Model file for the job. Use its own axes, mm. A direction names the side the tool comes from. Coordinates: 2 decimals unless noted, no trailing zeros. Order: outer loops, then holes, each group sorted by start corner. A loop starts at its lowest first (then second) coordinate and runs counter-clockwise, first axis right, second up.
from build123d import *

# Parameters (mm, degrees)
SKETCH1_R                                        = 28.448
EXTRUDE1_DEPTH                                   = 7.9375
CBORE_FOR_1_4_SOCKET_HEAD_CAP_SCREW1_D           = 6.7564
CBORE_FOR_1_4_SOCKET_HEAD_CAP_SCREW1_DEPTH       = 9.525
CBORE_FOR_1_4_SOCKET_HEAD_CAP_SCREW1_CBORE_D     = 11.1125
CBORE_FOR_1_4_SOCKET_HEAD_CAP_SCREW1_CBORE_DEPTH = 6.35
F_1_4_20_TAPPED_HOLE1_D                          = 5.1054
CBORE_FOR_1_4_SOCKET_HEAD_CAP_SCREW3_D           = 6.7564
CBORE_FOR_1_4_SOCKET_HEAD_CAP_SCREW3_DEPTH       = 9.525
CBORE_FOR_1_4_SOCKET_HEAD_CAP_SCREW3_CBORE_D     = 11.1125
CBORE_FOR_1_4_SOCKET_HEAD_CAP_SCREW3_CBORE_DEPTH = 6.35
F_1_4_20_TAPPED_HOLE4_D                          = 5.1054
CBORE_FOR_1_4_SOCKET_HEAD_CAP_SCREW4_D           = 6.7564
CBORE_FOR_1_4_SOCKET_HEAD_CAP_SCREW4_DEPTH       = 9.525
CBORE_FOR_1_4_SOCKET_HEAD_CAP_SCREW4_CBORE_D     = 11.1125
CBORE_FOR_1_4_SOCKET_HEAD_CAP_SCREW4_CBORE_DEPTH = 6.35
F_1_4_20_TAPPED_HOLE5_D                          = 5.1054
F_1_4_20_TAPPED_HOLE5_DEPTH                      = 9.525
CBORE_FOR_1_4_SOCKET_HEAD_CAP_SCREW5_D           = 6.7564
CBORE_FOR_1_4_SOCKET_HEAD_CAP_SCREW5_DEPTH       = 9.525
CBORE_FOR_1_4_SOCKET_HEAD_CAP_SCREW5_CBORE_D     = 11.1125
CBORE_FOR_1_4_SOCKET_HEAD_CAP_SCREW5_CBORE_DEPTH = 6.35
F_1_4_20_TAPPED_HOLE6_D                          = 5.1054
F_1_4_20_TAPPED_HOLE6_DEPTH                      = 9.525
FILLET1_R                                        = 3.175


with BuildPart() as part:
    # Sketch1 → Extrude1 (new, symmetric)
    with BuildSketch(Plane.XY):
        with BuildLine():
            Line((-39.6875, 76.2), (-39.6875, 0))
            ThreePointArc((-39.6875, 0), (-32.485618813, -22.798733003), (-13.49375, -37.323134477))
            Line((-13.49375, -37.323134477), (-13.49375, -56.373134477))
            Line((-13.49375, -56.373134477), (-3.96875, -56.373134477))
            Line((-3.96875, -56.373134477), (-3.96875, -36.296166184))
            ThreePointArc((-3.96875, -36.296166184), (0, 36.5125), (3.96875, -36.296166184))
            Line((3.96875, -36.296166184), (3.96875, -56.373134477))
            Line((3.96875, -56.373134477), (13.49375, -56.373134477))
            Line((13.49375, -56.373134477), (13.49375, -37.323134477))
            ThreePointArc((13.49375, -37.323134477), (15.940663019, -36.345466275), (18.317307692, -35.207582921))
            Line((18.317307692, -35.207582921), (46.483374029, -20.553736767))
            Line((46.483374029, -20.553736767), (55.275681722, -37.45337657))
            Line((55.275681722, -37.45337657), (63.725501623, -33.057222723))
            Line((63.725501623, -33.057222723), (54.93319393, -16.157582921))
            Line((54.93319393, -16.157582921), (31.487040084, 28.908123218))
            ThreePointArc((31.487040084, 28.908123218), (33.176067607, 34.260612279), (38.528556668, 32.571584756))
            Line((38.528556668, 32.571584756), (61.974710515, -12.494121383))
            Line((61.974710515, -12.494121383), (70.767018207, -29.393761185))
            Line((70.767018207, -29.393761185), (79.216838108, -24.997607339))
            Line((79.216838108, -24.997607339), (70.424530416, -8.097967537))
            Line((70.424530416, -8.097967537), (91.549080168, 2.892417079))
            ThreePointArc((91.549080168, 2.892417079), (112.919272476, 38.1), (91.549080168, 73.307582921))
            Line((91.549080168, 73.307582921), (70.424530416, 84.297967537))
            Line((70.424530416, 84.297967537), (79.216838108, 101.197607339))
            Line((79.216838108, 101.197607339), (70.767018207, 105.593761185))
            Line((70.767018207, 105.593761185), (61.974710515, 88.694121383))
            Line((61.974710515, 88.694121383), (38.528556668, 43.628415244))
            ThreePointArc((38.528556668, 43.628415244), (33.176067607, 41.939387721), (31.487040084, 47.291876782))
            Line((31.487040084, 47.291876782), (54.93319393, 92.357582921))
            Line((54.93319393, 92.357582921), (63.725501623, 109.257222723))
            Line((63.725501623, 109.257222723), (55.275681722, 113.65337657))
            Line((55.275681722, 113.65337657), (46.483374029, 96.753736767))
            Line((46.483374029, 96.753736767), (18.317307692, 111.407582921))
            ThreePointArc((18.317307692, 111.407582921), (15.940663019, 112.545466275), (13.49375, 113.523134477))
            Line((13.49375, 113.523134477), (13.49375, 132.573134477))
            Line((13.49375, 132.573134477), (3.96875, 132.573134477))
            Line((3.96875, 132.573134477), (3.96875, 112.496166184))
            ThreePointArc((3.96875, 112.496166184), (0, 39.6875), (-3.96875, 112.496166184))
            Line((-3.96875, 112.496166184), (-3.96875, 132.573134477))
            Line((-3.96875, 132.573134477), (-13.49375, 132.573134477))
            Line((-13.49375, 132.573134477), (-13.49375, 113.523134477))
            ThreePointArc((-13.49375, 113.523134477), (-32.485618813, 98.998733003), (-39.6875, 76.2))
        make_face()
        with Locations((73.231772476, 38.1)):
            Circle(SKETCH1_R, mode=Mode.SUBTRACT)
    extrude(amount=EXTRUDE1_DEPTH, both=True)

    # CBORE for 1/4 Socket Head Cap Screw1
    with Locations(Plane(origin=(13.49375, 0, 0), x_dir=(0, 0, -1), z_dir=(1, 0, 0))):
        with Locations((0, 123.048134477)):
            CounterBoreHole(CBORE_FOR_1_4_SOCKET_HEAD_CAP_SCREW1_D / 2, CBORE_FOR_1_4_SOCKET_HEAD_CAP_SCREW1_CBORE_D / 2, CBORE_FOR_1_4_SOCKET_HEAD_CAP_SCREW1_CBORE_DEPTH, depth=CBORE_FOR_1_4_SOCKET_HEAD_CAP_SCREW1_DEPTH)

    # 1/4-20 Tapped Hole1 (through all)
    with Locations(Plane(origin=(-3.96875, 0, 0), x_dir=(0, 0, -1), z_dir=(1, 0, 0))):
        with Locations((0, 123.048134477)):
            Hole(F_1_4_20_TAPPED_HOLE1_D / 2)

    # CBORE for 1/4 Socket Head Cap Screw3
    with Locations(Plane(origin=(13.49375, 0, 0), x_dir=(0, 0, -1), z_dir=(1, 0, 0))):
        with Locations((0, -46.848134477)):
            CounterBoreHole(CBORE_FOR_1_4_SOCKET_HEAD_CAP_SCREW3_D / 2, CBORE_FOR_1_4_SOCKET_HEAD_CAP_SCREW3_CBORE_D / 2, CBORE_FOR_1_4_SOCKET_HEAD_CAP_SCREW3_CBORE_DEPTH, depth=CBORE_FOR_1_4_SOCKET_HEAD_CAP_SCREW3_DEPTH)

    # 1/4-20 Tapped Hole4 (through all)
    with Locations(Plane(origin=(-3.96875, 0, 0), x_dir=(0, 0, -1), z_dir=(1, 0, 0))):
        with Locations((0, -46.848134477)):
            Hole(F_1_4_20_TAPPED_HOLE4_D / 2)

    # CBORE for 1/4 Socket Head Cap Screw4
    with Locations(Plane(origin=(20.907887704, -10.877662722, 0), x_dir=(0, 0, -1), z_dir=(0.8871201995900625, -0.46153846153845923, 0))):
        with Locations((0, 116.811059209)):
            CounterBoreHole(CBORE_FOR_1_4_SOCKET_HEAD_CAP_SCREW4_D / 2, CBORE_FOR_1_4_SOCKET_HEAD_CAP_SCREW4_CBORE_D / 2, CBORE_FOR_1_4_SOCKET_HEAD_CAP_SCREW4_CBORE_DEPTH, depth=CBORE_FOR_1_4_SOCKET_HEAD_CAP_SCREW4_DEPTH)

    # 1/4-20 Tapped Hole5
    with Locations(Plane(origin=(5.416551219, -2.818047337, 0), x_dir=(0, 0, -1), z_dir=(0.8871201995900618, -0.4615384615384606, 0))):
        with Locations((0, 116.811059209)):
            Hole(F_1_4_20_TAPPED_HOLE5_D / 2, depth=F_1_4_20_TAPPED_HOLE5_DEPTH)

    # CBORE for 1/4 Socket Head Cap Screw5
    with Locations(Plane(origin=(52.107222723, 27.109615385, 0), x_dir=(0, 0, -1), z_dir=(0.8871201995900624, 0.46153846153845934, 0))):
        with Locations((0, -49.2125)):
            CounterBoreHole(CBORE_FOR_1_4_SOCKET_HEAD_CAP_SCREW5_D / 2, CBORE_FOR_1_4_SOCKET_HEAD_CAP_SCREW5_CBORE_D / 2, CBORE_FOR_1_4_SOCKET_HEAD_CAP_SCREW5_CBORE_DEPTH, depth=CBORE_FOR_1_4_SOCKET_HEAD_CAP_SCREW5_DEPTH)

    # 1/4-20 Tapped Hole6
    with Locations(Plane(origin=(36.615886238, 19.05, 0), x_dir=(0, 0, -1), z_dir=(0.8871201995900614, 0.4615384615384613, 0))):
        with Locations((0, -49.2125)):
            Hole(F_1_4_20_TAPPED_HOLE6_D / 2, depth=F_1_4_20_TAPPED_HOLE6_DEPTH)

    # Fillet1
    fillet1_edges = [part.edges().sort_by_distance(p)[0] for p in [
        (-13.49375, 113.523134477, 0),
        (13.49375, 113.523134477, 0),
        (46.483374029, 96.753736767, 0),
        (70.424530416, 84.297967537, 0),
        (70.424530416, -8.097967537, 0),
        (46.483374029, -20.553736767, 0),
        (13.49375, -37.323134477, 0),
        (-13.49375, -37.323134477, 0),
    ]]
    fillet(fillet1_edges, radius=FILLET1_R)


solid = part.part
Q1. Which spindle directions (+Z, -Z, +X, -X, +Y, -Y) get a long thin tool onto all of the face, cutting with end or side? Do faces 1 (the face through (-3.969, -44, 0)), 2 (the face through (77.23, -21.18, 3.64)), 3 (the face through (7.144, 123, -4)), 4 (the face through (44.81, 39.35, -0.11)). Say none if no direction does.
Established:
face 1: +Z, -Z, -Y
face 2: +Z, -Z, +X
face 3: +X
face 4: +Z, -Z
Q2. Cut at B-B, the plane y = 69.5. List the corners of the cut face in (x, z), plus the area to 3 significant figures.
Established:
outline: (-39.69, -7.94) - (-35.89, -7.94) - (-35.89, 7.94) - (-39.69, 7.94) - close; (35.89, -7.94) - (43.04, -7.94) - (43.04, 7.94) - (35.89, 7.94) - close; (51.99, -7.94) - (97.5, -7.94) - (97.5, 7.94) - (51.99, 7.94) - close
area: 896 mm2
Q3. Probe line 1 (Y direction, x = -8.5, z = -4.5); line 2 (Y direction, x = 76.5, z = 1.5); line 3 (X direction, y = 71.5, z = -5.25). List the from-to ranges inside material, lowest first.
Established:
line 1: y = -56.37 to -35.51, 35.51 to 40.69, 111.71 to 132.57
line 2: y = -26.41 to -21.7, -4.94 to 9.84, 66.36 to 81.14, 97.9 to 102.61
line 3: x = -39.69 to -36.21, 36.21 to 44.08, 53.03 to 94.67
Q4. Cut at C-C, the plane x = 96. List the corners of the cut face in (y, z).
Established:
outline: (5.59, -7.94) - (21.04, -7.94) - (21.04, 7.94) - (5.59, 7.94) - close; (55.16, -7.94) - (70.61, -7.94) - (70.61, 7.94) - (55.16, 7.94) - close
Q5. Cut at A-A, the plane x = -26.5. List the corners of the cut face in (y, z), plus the area to 3 significant figures.
Established:
outline: (-29.54, -7.94) - (-25.12, -7.94) - (-25.12, 7.94) - (-29.54, 7.94) - close; (25.12, -7.94) - (51.08, -7.94) - (51.08, 7.94) - (25.12, 7.94) - close; (101.32, -7.94) - (105.74, -7.94) - (105.74, 7.94) - (101.32, 7.94) - close
area: 553 mm2
Q6. Drop flat-ended pins along their axis: P1, Ø2, axis at x = 39.5, z = -3.5, coming from the +Y side; P2, Ø5.5, axis at y = 123.05, z = 0, coming from the -X side; P3, Ø9, axis at y = 123.05, z = 0, coming from the +X side. Give the stop position or say it passes through.
Established:
P1: stops at y = 100.91
P2: stops at x = -13.49
P3: stops at x = 7.14
Q7. Cut at D-D, the plane z = 0. Count the separate pieces of the cut face and the enclosed holes in it, plus the area to 3 significant figures.
Established:
separate pieces: 9
enclosed holes: 1
area: 6,340 mm2
Q8. Mould opens along Y. For faces 5 (the face through (52.48, 108.28, 0.11)), 6 (the face through (-13.494, 126, 0)), 7 (the face through (77.13, 97.19, 3.64)) say: pulls with the +Y half, pulls with the -Y half, needs draft (parallel to the pull), parting line crosses it, or undercut.
Established:
face 5: pulls with the +Y half
face 6: needs draft
face 7: undercut
